Here's how the part is built. I have some questions about the finished solid (model axes, mm). Face numbers are marked on the shaded views. A direction names the side the tool comes from. Coordinates: 2 decimals unless noted, no trailing zeros. Write each loop counter-clockwise with the first axis right and the second up, starting at its lowest first coordinate (ties: lowest second). Pieces come first, ordered by that corner, then holes. Notation, with made-up numbers: M 82.5,14.25 L 122.5,14.25 A17 cw 122.5,22.25 Z; hole C -10.5,66.25 d3. An arc over 180 degrees is marked long. Use a Markdown table: item, result.
```python
from build123d import *

# Parameters (mm, degrees)
SKETCH_1_R      = 6.25
EXTRUDE_2_DEPTH = 10
SHELL_1_T       = -2
SKETCH_2_R      = 2.75
EXTRUDE_3_DEPTH = 10


with BuildPart() as part:
    # 草图1 → 凸台-拉伸2 (new body)
    with BuildSketch(Plane(origin=(0, 0, 0), x_dir=(1, 0, 0), z_dir=(0, 1, 0))):
        with Locations(Location((0, 0, 0), (0, 0, 270))):
            Circle(SKETCH_1_R)
    extrude(amount=EXTRUDE_2_DEPTH)

    # 抽壳1
    shell_1_openings = [part.faces().sort_by_distance(p)[0] for p in [
        (0, 10, 0),
    ]]
    offset(amount=SHELL_1_T, openings=shell_1_openings, kind=Kind.INTERSECTION)

    # 草图2 → 凸台-拉伸3 (add)
    with BuildSketch(Plane(origin=(0, 2, 0), x_dir=(1, 0, 0), z_dir=(0, 1, 0))):
        with Locations(Location((0, 0, 0), (0, 0, 270))):
            Circle(SKETCH_2_R)
    extrude(amount=EXTRUDE_3_DEPTH)


solid = part.part
```
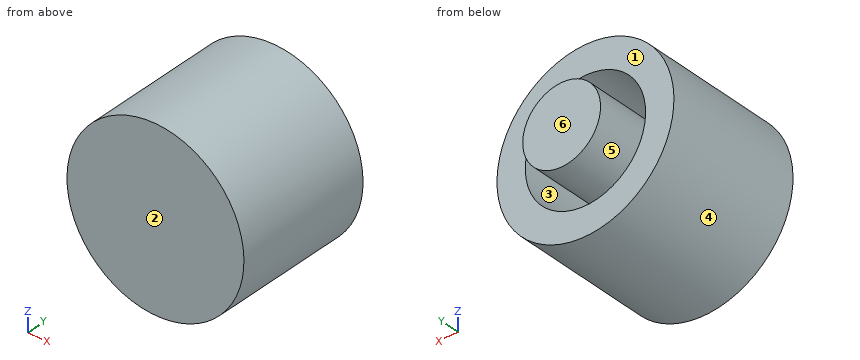
1. Suppose I cut it at D-D on y = 11.5. Write out the boundary of the cut face in (x, z).
Answers follow:
| item | result |
|---|---|
| outline | C 0,0 d5.5 |
2. Will these pins go through, and if not, where does the flat tip stop? pin 1 Ø5 at (x, z) = (-1, 5) entering from -Y; pin 2 Ø1.5 at (x, y) = (-1.5, 5) entering from +Z; pin 3 Ø3 at (x, y) = (-4, 8.5) entering from +Z.
Answers follow:
| item | result |
|---|---|
| pin 1 | stops at y = 0 |
| pin 2 | stops at z = 6.2 |
| pin 3 | stops at z = 5.73 |
3. Which directions (+Z, -Z, +X, -X, +Y, -Y) give clear straight access to the entire face, cutting with the end or side of a thin tool? Please do the marked faces 1 and 2.
Answers follow:
| item | result |
|---|---|
| face 1 | +Y |
| face 2 | +Z, -Z, +X, -X, -Y |
4. I need wall thicknesses on probe 1 along X at (y, z) = (5.75, 0); probe 2 along X at (y, z) = (7, 1.5); probe 3 along Z at (x, y) = (-0.25, 5.5) (3 decimals). Which ranges of each line are inside material? Lowest first, please.
Answers follow:
| item | result |
|---|---|
| probe 1 | x = -6.25 to -4.25, -2.75 to 2.75, 4.25 to 6.25 |
| probe 2 | x = -6.07 to -3.98, -2.3 to 2.3, 3.98 to 6.07 |
| probe 3 | z = -6.245 to -4.243, -2.739 to 2.739, 4.243 to 6.245 |
5. We'd pull the mould along X, two halves only. Please class the marked faces 3, 4, 5 and 6: +X half, -X half, draft (parallel to the pull), parting line (faces both ways), or undercut.
Answers follow:
| item | result |
|---|---|
| face 3 | undercut |
| face 4 | parting line |
| face 5 | undercut |
| face 6 | draft |
6. Suppose I cut it at C-C on z = 0. Write out the boundary of the cut face in (x, y).
Answers follow:
| item | result |
|---|---|
| outline | M -6.25,0 L 6.25,0 L 6.25,10 L 4.25,10 L 4.25,2 L 2.75,2 L 2.75,12 L -2.75,12 L -2.75,2 L -4.25,2 L -4.25,10 L -6.25,10 Z |
7. Suppose I cut it at A-A on y = 2.75. Write out the boundary of the cut face in (x, z).
Answers follow:
| item | result |
|---|---|
| outline | C 0,0 d12.5; C 0,0 d5.5; hole C 0,0 d8.5 |
8. Suppose I cut it at B-B on x = 0. Write out the boundary of the cut face in (y, z), and give its area (3 significant figures).
Answers follow:
| item | result |
|---|---|
| outline | M 0,-6.25 L 10,-6.25 L 10,-4.25 L 2,-4.25 L 2,-2.75 L 12,-2.75 L 12,2.75 L 2,2.75 L 2,4.25 L 10,4.25 L 10,6.25 L 0,6.25 Z |
| area | 112 mm2 |
